Can you work these out from the model? Positions are in its coordinate system, mm. A direction names the side the tool comes from. Round coordinates to 2 decimals unless told otherwise and drop trailing zeros. Write each loop counter-clockwise with the first axis right and the second up, starting at its lowest first coordinate (ties: lowest second). Pieces come first, ordered by that corner, then holes. Notation, with made-up numbers: M 89,66.5 L 142,66.5 A12 ccw 142,84.5 Z; hole C 21.25,-0.75 d2. An arc over 180 degrees is marked long. Answer as a JSON object with one key per item and string values. Group by question number.
1) Suppose I cut it at A-A, the plane x = 26.5. Write out the boundary of the cut face in (y, z).
2) I'm going to push flat-ended pins straight in: pin 1 Ø2.5 at (y, z) = (2, 3.5) entering from -X; pin 2 Ø1.6 at (x, z) = (2, 3.5) entering from +Y; pin 3 Ø2.5 at (y, z) = (135.5, 2) entering from -X. Where does each tip first touch, or does it pass through?
3) Suppose I cut it at C-C, the plane x = 9. Write out the boundary of the cut face in (y, z), and give its area (3 significant figures).
4) If we mould it in two halves opening along X, with no side actions, what happens to faces 5 (the flat face through (34, 150, 3)), 6 (the flat face through (28, 295.35, 3)), 7 (the flat face through (0, 265, 3)), 8 (the flat face through (16.198, 82, 3))? For each: +X half, -X half, draft (parallel to the pull), parting line (faces both ways), or undercut.
5) Suppose I cut it at B-B, the plane y = 213.5. Write out the boundary of the cut face in (x, z), and give its area (3 significant figures).
6) On a 3-axis mill with a long thin cutter (end or side, diameter ignored), from which of +Z, -Z, +X, -X, +Y, -Y can I reach the whole of each face in a straight line? I mean faces 1 (the flat face through (27, 105.35, 3)), 2 (the flat face through (5.35, 15, 3)), 3 (the flat face through (8, 295.35, 3)), 4 (the flat face through (5.35, 152, 3)). Say none if no direction works.
7) Please list where these lines run through material, in increasing order: L1, parallel to Y at x = 26, z = 4.8; L2, parallel to Y at x = 21, z = 0.7; L3, parallel to Y at x = 20, z = 4.1. Write a range as [from, to].
from build123d import *

# Parameters (mm, degrees)
BOSS_EXTRUDE1_DEPTH = 5.35


with BuildPart() as part:
    # Model → Boss-Extrude1 (new body)
    with BuildSketch(Plane.XY):
        Polygon((0, 25.350004435), (5.350001156, 25.350004435), (5.350001156, 5.350008607), (11.500000954, 5.350008607), (11.500000954, 0), (21.50000073, 0), (21.50000073, 5.350008607), (34.000000916, 5.350008607), (34.000000916, 105.350002646), (19.675000687, 105.350002646), (19.675000687, 110.700011253), (34.000000916, 110.700011253), (34.000000916, 190.000005066), (19.675000687, 190.000005066), (19.675000687, 195.350006223), (34.000000916, 195.350006223), (34.000000916, 295.350007713), (21.50000073, 295.350007713), (21.50000073, 300.700008869), (11.500000954, 300.700008869), (11.500000954, 295.350007713), (5.350001156, 295.350007713), (5.350001156, 275.35000816), (0, 275.35000816), (0, 255.350007676), (5.350001156, 255.350007676), (5.350001156, 45.350000262), (0, 45.350000262), align=None)
        with BuildLine():
            Line((20.197596634, 77.811388135), (20.197596634, 85.811391473))
            ThreePointArc((20.197596634, 85.811391473), (19.904704132, 86.518499564), (19.197596634, 86.811393499))
            Line((19.197596634, 86.811393499), (17.197596841, 86.811393499))
            ThreePointArc((17.197596841, 86.811393499), (16.490489953, 86.518500339), (16.197596677, 85.811393499))
            Line((16.197596677, 85.811393499), (16.197596677, 77.811390161))
            ThreePointArc((16.197596677, 77.811390161), (16.490489179, 77.10428207), (17.197596677, 76.811388135))
            Line((17.197596677, 76.811388135), (19.197596703, 76.811388135))
            ThreePointArc((19.197596703, 76.811388135), (19.904703439, 77.104281378), (20.197596634, 77.811388135))
        make_face(mode=Mode.SUBTRACT)
    extrude(amount=BOSS_EXTRUDE1_DEPTH)


solid = part.part
Results:
{
 "1": {"outline": "M 5.35,0 L 105.35,0 L 105.35,5.35 L 5.35,5.35 Z; M 110.7,0 L 190,0 L 190,5.35 L 110.7,5.35 Z; M 195.35,0 L 295.35,0 L 295.35,5.35 L 195.35,5.35 Z"},
 "2": {"pin 1": "x = 11.5", "pin 2": "y = 275.35", "pin 3": "x = 5.35"},
 "3": {"outline": "M 5.35,0 L 295.35,0 L 295.35,5.35 L 5.35,5.35 Z", "area": "1,550 mm^2"},
 "4": {"face 5": "+X half", "face 6": "draft", "face 7": "-X half", "face 8": "undercut"},
 "5": {"outline": "M 5.35,0 L 34,0 L 34,5.35 L 5.35,5.35 Z", "area": "153 mm^2"},
 "6": {"face 1": "+Z, -Z, +X", "face 2": "+Z, -Z, -X, -Y", "face 3": "+Z, -Z, -X, +Y", "face 4": "+Z, -Z, -X"},
 "7": {"L1": "[5.35, 105.35], [110.7, 190], [195.35, 295.35]", "L2": "[0, 105.35], [110.7, 190], [195.35, 300.7]", "L3": "[0, 77.21], [86.41, 105.35], [110.7, 190], [195.35, 300.7]"}
}
